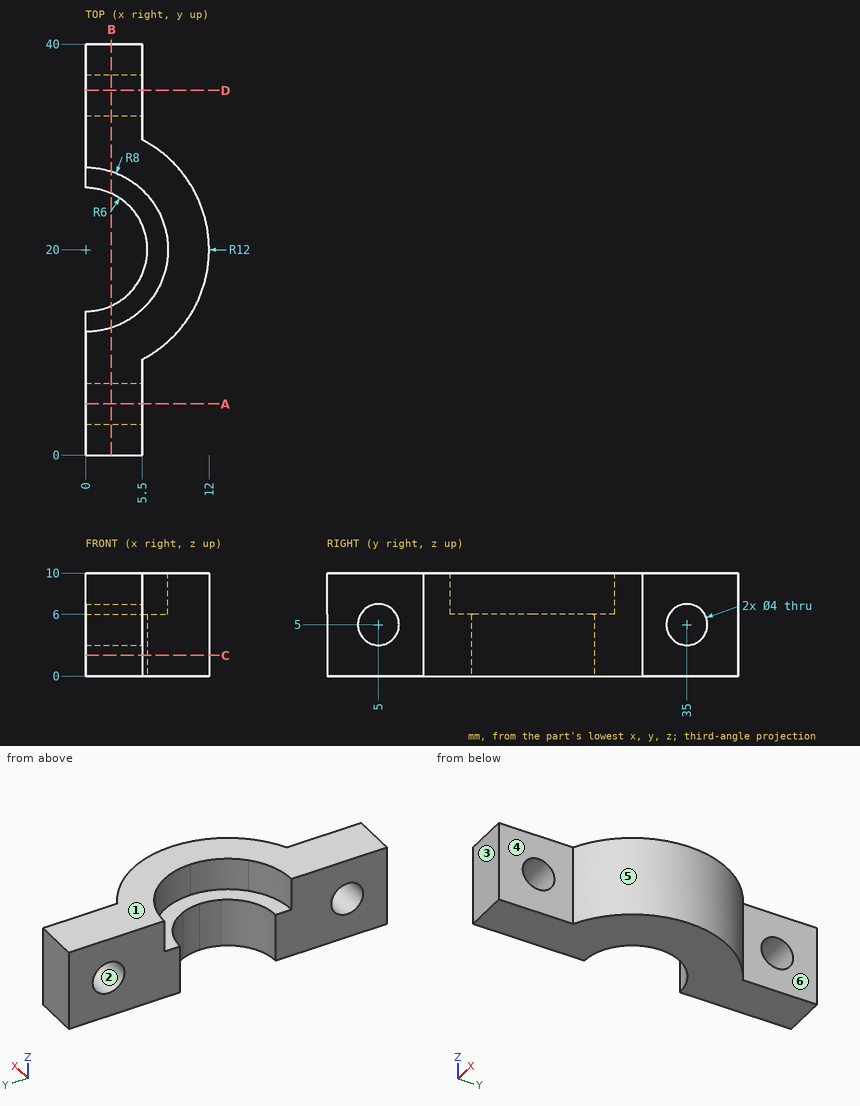
Drawing for the job (mm, zero at the part's lowest x, y, z). A direction names the side the tool comes from. Round coordinates to 2 decimals unless told otherwise and drop trailing zeros. Loops run counter-clockwise (first coordinate to the right, second up) from the corner with the lowest first, then second, coordinate; pieces in that order, holes last. Notation, with made-up numbers: (81, 53.25) -> (104, 53.25) arc R11 ccw to (104, 58.25) -> close; hole circle Ø1 at (66.25, -23). An arc over 180 degrees is marked (long way). Use one line per item in the form item = value. Start each with the question number.
Item 1: Band-saw the part on C-C (z = 2). List the corners of the cut face in (x, y).
Item 2: Drop flat-ended pins along their axis: pin 1 Ø2 at (y, z) = (24.5, 8) entering from -X; pin 2 Ø1 at (y, z) = (10, 7) entering from +X; pin 3 Ø4 at (y, z) = (9.5, 5.5) entering from +X. Give the stop position or say it passes through.
Item 3: Band-saw the part on B-B (x = 2.5). List the corners of the cut face in (y, z).
Item 4: Band-saw the part on D-D (y = 35.5). List the corners of the cut face in (x, z), plus the area to 3 significant figures.
Item 5: Tool access for the marked faces 4, 5 and 6: list every direction of +Z, -Z, +X, -X, +Y, -Y with a clear straight run to the whole face (end or side of a thin tool).
Item 6: Band-saw the part on A-A (y = 5). List the corners of the cut face in (x, z).
Item 7: Drill centre lines: line 1 along Z through (x, y) = (1.9, 35); line 2 along Y through (x, z) = (3.5, 4.5); line 3 along Y through (x, z) = (6.75, 7.5). Where is each one in solid material? Low to high.
Item 8: Two-plate mould, pull along Y, no slides. Class the marked faces 1, 2 and 3: released by +Y, released by -Y, zero draft, split by the parting line, or undercut.
Data:
q1.outline = (0, 0) -> (5.5, 0) -> (5.5, 9.33) arc R12 ccw to (5.5, 30.67) -> (5.5, 40) -> (0, 40) -> (0, 26) arc R6 cw to (0, 14) -> close
q2.pin_1 = 5.81
q2.pin_2 = 7.33
q2.pin_3 = 8.47
q3.outline = (0, 0) -> (14.55, 0) -> (14.55, 6) -> (12.4, 6) -> (12.4, 10) -> (0, 10) -> close; (25.45, 0) -> (40, 0) -> (40, 10) -> (27.6, 10) -> (27.6, 6) -> (25.45, 6) -> close; hole circle Ø4 at (5, 5); hole circle Ø4 at (35, 5)
q4.outline = (0, 0) -> (5.5, 0) -> (5.5, 3.06) -> (0, 3.06) -> close; (0, 6.94) -> (5.5, 6.94) -> (5.5, 10) -> (0, 10) -> close
q4.area = 33.7 mm^2
q5.face_4 = +Z, -Z, +X, -Y
q5.face_5 = +Z, -Z, +X
q5.face_6 = +Z, -Z, +X, +Y
q6.outline = (0, 0) -> (5.5, 0) -> (5.5, 3) -> (0, 3) -> close; (0, 7) -> (5.5, 7) -> (5.5, 10) -> (0, 10) -> close
q7.line_1 = 0 to 3, 7 to 10
q7.line_2 = 0 to 3.06, 6.94 to 15.13, 24.87 to 33.06, 36.94 to 40
q7.line_3 = 10.08 to 15.71, 24.29 to 29.92
q8.face_1 = zero draft
q8.face_2 = undercut
q8.face_3 = released by -Y
